Could you check a few things on this model? Use its own coordinates, in mm. Round coordinates to 2 decimals unless told otherwise and drop trailing zeros. Loops run counter-clockwise (first coordinate to the right, second up) from the corner with the lowest first, then second, coordinate; pieces in that order, holes last. Notation, with made-up numbers: (68, 33.5) -> (72, 33.5) arc R27 ccw to (72, 56.5) -> close; hole circle Ø6 at (63.25, 84). An arc over 180 degrees is marked (long way). One line per item, written item: value.
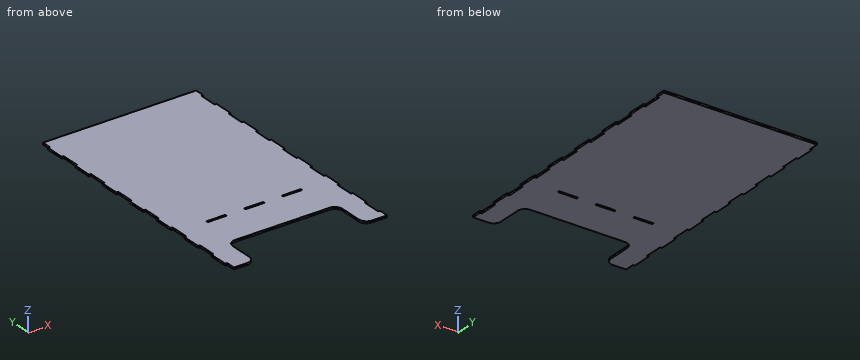
```python
from build123d import *

# Parameters (mm, degrees)
AUFSATZ_LINEAR_AUSTRAGEN1_DEPTH = 5
SKIZZE2_W                       = 50.3
SKIZZE2_H                       = 4.8
SCHNITT_LINEAR_AUSTRAGEN1_DEPTH = 5
LINEARES_MUSTER1_COUNT          = 3
LINEARES_MUSTER1_PITCH          = 99.9
SKIZZE3_W                       = 92.912444059
SKIZZE3_H                       = 49.6
SCHNITT_LINEAR_AUSTRAGEN2_DEPTH = 5
LINEARES_MUSTER2_COUNT          = 8
LINEARES_MUSTER2_PITCH          = 99.9
SKIZZE4_W                       = 86.468004991
SKIZZE4_H                       = 49.6
SCHNITT_LINEAR_AUSTRAGEN4_DEPTH = 5
LINEARES_MUSTER3_COUNT          = 7
LINEARES_MUSTER3_PITCH          = 99.9


with BuildPart() as part:
    # Skizze1 → Aufsatz-Linear austragen1 (new body)
    with BuildSketch(Plane.XY):
        with BuildLine():
            Line((0, 0), (0, 700))
            Line((0, 700), (410, 700))
            Line((410, 700), (410, 0))
            Line((410, 0), (370, 0))
            ThreePointArc((370, 0), (355.857864376, 5.857864376), (350, 20))
            Line((350, 20), (350, 80))
            ThreePointArc((350, 80), (344.142135624, 94.142135624), (330, 100))
            Line((330, 100), (80, 100))
            ThreePointArc((80, 100), (65.857864376, 94.142135624), (60, 80))
            Line((60, 80), (60, 20))
            ThreePointArc((60, 20), (54.142135624, 5.857864376), (40, 0))
            Line((40, 0), (0, 0))
        make_face()
    extrude(amount=AUFSATZ_LINEAR_AUSTRAGEN1_DEPTH)

    # Skizze2 → Schnitt-Linear austragen1 (cut)
    with BuildSketch(Plane.XY.offset(5)):
        with Locations((105.1, 202.4)):
            Rectangle(SKIZZE2_W, SKIZZE2_H)
    schnitt_linear_austragen1 = extrude(amount=-SCHNITT_LINEAR_AUSTRAGEN1_DEPTH, mode=Mode.SUBTRACT)

    # Lineares Muster1: Schnitt-Linear austragen1 ×3
    with Locations(*[(i * LINEARES_MUSTER1_PITCH, 0, 0) for i in range(1, LINEARES_MUSTER1_COUNT)]):
        add(schnitt_linear_austragen1, mode=Mode.SUBTRACT)

    # Skizze3 → Schnitt-Linear austragen2 (cut)
    with BuildSketch(Plane.XY.offset(5)):
        with Locations((-41.45622203, 699.3)):
            Rectangle(SKIZZE3_W, SKIZZE3_H)
    schnitt_linear_austragen2 = extrude(amount=-SCHNITT_LINEAR_AUSTRAGEN2_DEPTH, mode=Mode.SUBTRACT)

    # Lineares Muster2: Schnitt-Linear austragen2 ×8
    with Locations(*[(0, -i * LINEARES_MUSTER2_PITCH, 0) for i in range(1, LINEARES_MUSTER2_COUNT)]):
        add(schnitt_linear_austragen2, mode=Mode.SUBTRACT)

    # Skizze4 → Schnitt-Linear austragen4 (cut)
    with BuildSketch(Plane.XY.offset(5)):
        with Locations((448.234002496, 649.7)):
            Rectangle(SKIZZE4_W, SKIZZE4_H)
    schnitt_linear_austragen4 = extrude(amount=-SCHNITT_LINEAR_AUSTRAGEN4_DEPTH, mode=Mode.SUBTRACT)

    # Lineares Muster3: Schnitt-Linear austragen4 ×7
    with Locations(*[(0, -i * LINEARES_MUSTER3_PITCH, 0) for i in range(1, LINEARES_MUSTER3_COUNT)]):
        add(schnitt_linear_austragen4, mode=Mode.SUBTRACT)


solid = part.part
```
(1) For pin 1 Ø2.5 at (y, z) = (197.5, 2.5) entering from -X; pin 2 Ø1.5 at (x, z) = (315.5, 2) entering from -Y; pin 3 Ø2.5 at (y, z) = (250, 3.5) entering from +X, each with a flat end and sliding along its axis, tell me the tip position at first contact or that it passes through.
Results below:
pin 1: stops at x = 5
pin 2: stops at y = 100
pin 3: stops at x = 405
(2) Please list where these lines run through material, in increasing order: L1, parallel to Y at x = 312.5, z = 3.45; L2, parallel to X at y = 446.5, z = 3.35; L3, parallel to X at y = 524, z = 0.5.
Results below:
L1: y = 100 to 200, 204.8 to 700
L2: x = 0 to 405
L3: x = 5 to 410
(3) Imagine slicing it at C-C on x = 269. Write out the boundary of the cut face in (y, z), then the cut area to 3 significant figures.
Results below:
outline: (100, 0) -> (700, 0) -> (700, 5) -> (100, 5) -> close
area: 3,000 mm²
(4) Imagine slicing it at B-B on z = 2.1. Give the number of separate pieces and of enclosed holes in the cut face, then the cut area to 3 significant figures.
Results below:
separate pieces: 1
enclosed holes: 3
area: 254,000 mm²
(5) Imagine slicing it at A-A on y = 63.5. Write out the boundary of the cut face in (x, z).
Results below:
outline: (0, 0) -> (60, 0) -> (60, 5) -> (0, 5) -> close; (350, 0) -> (405, 0) -> (405, 5) -> (350, 5) -> close
(6) Imagine slicing it at D-D on x = 338. Write out the boundary of the cut face in (y, z).
Results below:
outline: (98.33, 0) -> (700, 0) -> (700, 5) -> (98.33, 5) -> close
